The drawing under review shows one solid part. Ordinate dimensions are in mm from its lowest x, y, z. A direction names the side the tool comes from. Give positions to 0.01 mm unless a question says otherwise; leave off trailing zeros. Loops run counter-clockwise (first coordinate to the right, second up) from the corner with the lowest first, then second, coordinate; pieces in that order, holes last. Notation, with made-up numbers: M 71.5,67.5 L 118.5,67.5 A17 cw 118.5,82.5 Z; hole C -33,-34 d6. An arc over 180 degrees is marked long. Write item = value, one per line. Start each with the question number.
1. We need section A-A on y = 10.16. Give the boundary of the cut face in (x, z), then the cut area to 3 significant figures.
2. Wall thickness on line 1 along Z through (x, y) = (6.25, 2.5); line 2 along X through (y, z) = (10.25, 50): over which ranges is each line inside the solid? List them lowest first. Write a range as from..to.
3. We need section C-C on z = 85. Give the boundary of the cut face in (x, y).
4. For the marked faces 1, 2 and 3, list the 3-axis set-ups (+Z, -Z, +X, -X, +Y, -Y) from which the entire face can be reached by the end or side of a thin tool; tool diameter is ignored.
5. For pin 1 (1 mm diameter, centred on x = 11.5, z = 43.5, fed in from -Y); pin 2 (4 mm diameter, centred on x = 3.5, y = 6, fed in from +Z); pin 3 (4 mm diameter, centred on x = 18, z = 47.5, fed in from +Y); pin 4 (6 mm diameter, centred on x = 6.5, z = 64, fed in from +Y), all flat-tipped, find the tip position at first contact; note any pin that passes through.
6. We need section D-D on z = 18. Give the boundary of the cut face in (x, y), then the cut area to 3 significant figures.
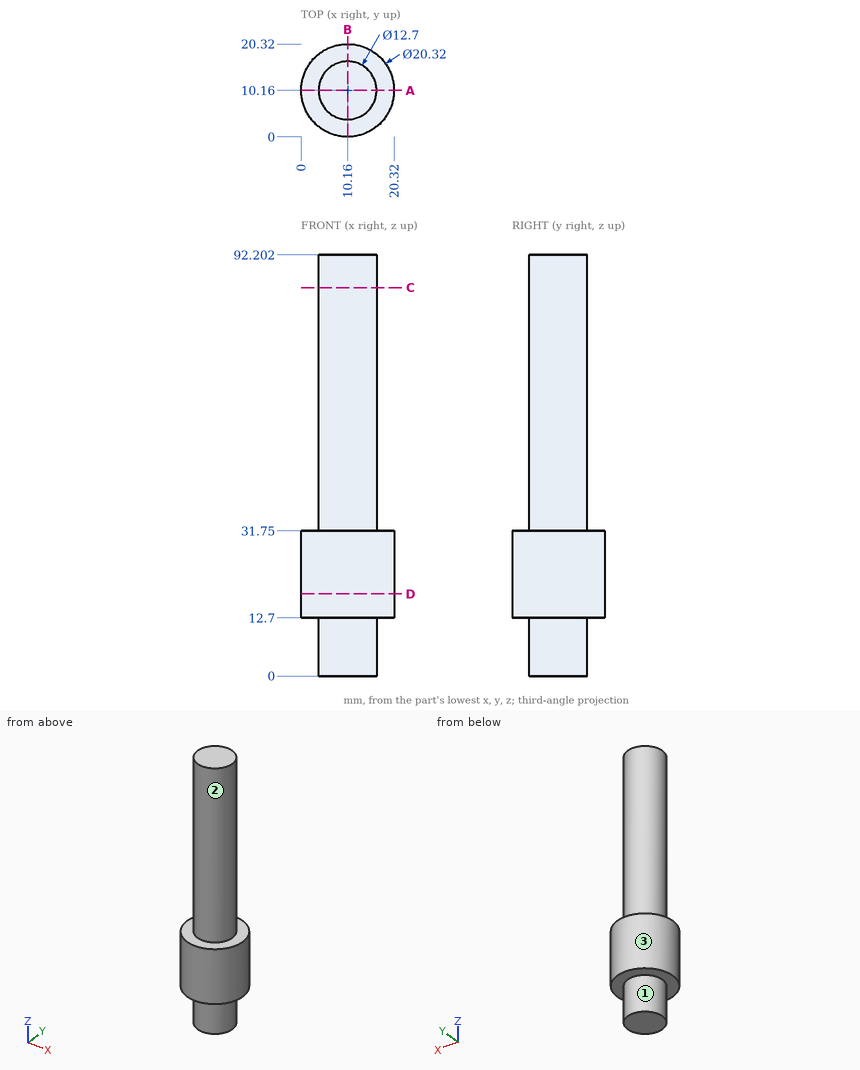
Final values:
q1.outline = M 0,12.7 L 3.81,12.7 L 3.81,0 L 16.51,0 L 16.51,12.7 L 20.32,12.7 L 20.32,31.75 L 16.51,31.75 L 16.51,92.2 L 3.81,92.2 L 3.81,31.75 L 0,31.75 Z
q1.area = 1,320 mm²
q2.line_1 = 12.7..31.75
q2.line_2 = 3.81..16.51
q3.outline = C 10.16,10.16 d12.7
q4.face_1 = -Z
q4.face_2 = +Z
q4.face_3 = +Z, -Z
q5.pin_1 = 3.87
q5.pin_2 = 92.2
q5.pin_3 = 12.65
q5.pin_4 = 16.48
q6.outline = C 10.16,10.16 d20.32
q6.area = 324 mm²
